Input: part model. Units: mm. Frame: model coordinates. Coordinates: 2 decimals unless noted, no trailing zeros. Order: outer loops, then holes, each group sorted by start corner. A loop starts at its lowest first (then second) coordinate and runs counter-clockwise, first axis right, second up. Notation, with made-up numbers: (70.5, -26.5) -> (89.5, -26.5) arc R34 cw to (89.5, 7.5) -> close; hole circle Ø2 at (9.25, 48). An arc over 180 degrees is marked (long way). Write each question's results on one line, items separated by ' | '.
```python
from build123d import *

# Parameters (mm, degrees)
F1_DEPTH = 3.175
F3_D     = 3.2512


with BuildPart() as f1:
    # F0 (on Front) → F1 (new body)
    with BuildSketch(Plane.XZ):
        with BuildLine():
            ThreePointArc((4.073034, -2.413141), (4.565934, -1.251041), (4.734222, 0))
            ThreePointArc((4.734222, 0), (4.514878, 1.424338), (3.87717, 2.716692))
            ThreePointArc((3.87717, 2.716692), (-4.730775, -0.180628), (4.073034, -2.413141))
        make_face()
        with BuildLine():
            ThreePointArc((3.87717, 2.716692), (4.514878, 1.424338), (4.734222, 0))
            ThreePointArc((4.734222, 0), (4.565934, -1.251041), (4.073034, -2.413141))
            Line((4.073034, -2.413141), (84.995226, -2.413141))
            ThreePointArc((84.995226, -2.413141), (84.335839, 0.180791), (85.191691, 2.716692))
            Line((85.191691, 2.716692), (3.87717, 2.716692))
        make_face()
        with BuildLine():
            ThreePointArc((93.780427, 0), (90.481081, 4.504076), (85.191691, 2.716692))
            ThreePointArc((85.191691, 2.716692), (84.335839, 0.180791), (84.995226, -2.413141))
            ThreePointArc((84.995226, -2.413141), (90.307663, -4.555299), (93.780427, 0))
        make_face()
    extrude(amount=F1_DEPTH)

    # F3 (through all)
    with Locations(Plane(origin=(0, 0, 0), x_dir=(1, 0, 0), z_dir=(0, 1, 0))):
        with Locations((0, 0), (89.366406, 0)):
            Hole(F3_D / 2)


solid = f1.part
```
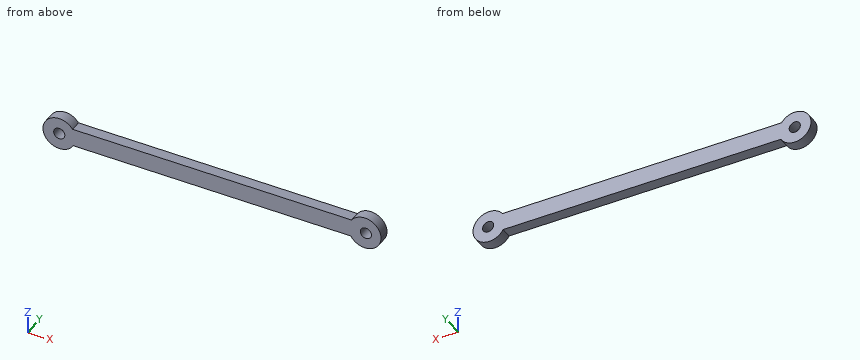
(1) Cut plane B-B, the plane y = -2.35. Return loops of the section in (x, z), plus the area to 3 significant figures.
Return value:
outline: (3.88, 2.72) arc R4.73 ccw (long way) to (4.07, -2.41) -> (85, -2.41) arc R4.72 ccw (long way) to (85.19, 2.72) -> close; hole circle Ø3.25 at (0, 0); hole circle Ø3.25 at (89.37, 0) | area: 535 mm2
(2) Cut plane A-A, the plane x = 0. Return loops of the section in (y, z) (3 decimals).
Return value:
outline: (-3.175, -4.734) -> (0, -4.734) -> (0, -1.626) -> (-3.175, -1.626) -> close; (-3.175, 1.626) -> (0, 1.626) -> (0, 4.734) -> (-3.175, 4.734) -> close
(3) Pin query (flat end, axial travel): P1, Ø1.6, axis at x = 33, y = -1.5, coming from the +Z side; P2, Ø1, axis at y = -0.5, z = 3, coming from the +X side. Return the tip coordinate at first contact, or that it passes through.
Return value:
P1: z = 2.72 | P2: x = 93.06
(4) Line query: line 1 along Z through (x, y) = (0, -1.55); line 2 along X through (y, z) = (-2.55, 1); line 3 along Z through (x, y) = (23, -2.85). Output: solid intervals per line, ascending. Write a range as from..to.
Return value:
line 1: -4.73..-1.63, 1.63..4.73 | line 2: -4.63..-1.28, 1.28..88.08, 90.65..93.67 | line 3: -2.41..2.72
(5) Cut plane C-C, the plane x = 55.5. Return loops of the section in (y, z) (3 decimals).
Return value:
outline: (-3.175, -2.413) -> (0, -2.413) -> (0, 2.717) -> (-3.175, 2.717) -> close
